Design review of the part built by this model. Coordinates are the model's own, in mm. Face numbers are marked on the shaded views. A direction names the side the tool comes from. Round coordinates to 2 decimals unless told otherwise and drop trailing zeros. Order: outer loops, then holes, each group sorted by start corner. A loop starts at its lowest first (then second) coordinate and runs counter-clockwise, first axis right, second up. Notation, with made-up numbers: (62.5, 89) - (110.5, 89) arc R37 ccw to (110.5, 127) - close; hole circle Ø2 at (75.5, 62.25). An arc over 180 degrees is marked (long way). Use CSV: the item, a comma, the result in double quotes.
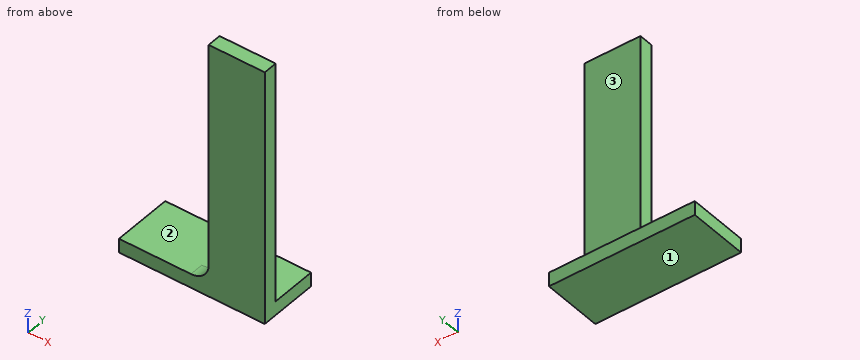
from build123d import *

# Parameters (mm, degrees)
SKETCH1_W      = 52
SKETCH1_H      = 21.25
EXTRUDE1_DEPTH = 5
SKETCH2_W      = 20
SKETCH2_H      = 5
EXTRUDE2_DEPTH = 86.5
FILLET1_R      = 6.35


with BuildPart() as part:
    # Sketch1 → Extrude1 (new body)
    with BuildSketch(Plane.XY):
        with Locations((26, -10.625)):
            Rectangle(SKETCH1_W, SKETCH1_H)
    extrude(amount=EXTRUDE1_DEPTH)

    # Sketch2 → Extrude2 (add)
    with BuildSketch(Plane.XY.offset(5)):
        with Locations((42, -18.75)):
            Rectangle(SKETCH2_W, SKETCH2_H)
    extrude(amount=EXTRUDE2_DEPTH)

    # Fillet1
    fillet1_edges = [part.edges().sort_by_distance(p)[0] for p in [
        (32, -18.75, 5),
    ]]
    fillet(fillet1_edges, radius=FILLET1_R)


solid = part.part
1) Insertion check: pin 1 Ø12 at (y, z) = (-14.5, 55.5) entering from -X; pin 2 Ø1.5 at (y, z) = (-16, 9.5) entering from -X; pin 3 Ø1 at (x, y) = (35.5, -7) entering from -Z; pin 4 Ø6.5 at (x, y) = (36, -12.5) entering from +Z. Each pin has a flat end and moves straight along its axis. Give the tip position at first contact, or say it passes through.
Data:
pin 1,"stops at x = 32"
pin 2,"stops at x = 31.46"
pin 3,"stops at z = 0"
pin 4,"stops at z = 5"
2) We need section B-B (x = 22). Give the boundary of the cut face in (y, z), then the cut area to 3 significant figures.
Data:
outline,"(-21.25, 0) - (0, 0) - (0, 5) - (-21.25, 5) - close"
area,"106 mm2"
3) For the marked faces 1, 2 and 3, list the 3-axis set-ups (+Z, -Z, +X, -X, +Y, -Y) from which the entire face can be reached by the end or side of a thin tool; tool diameter is ignored.
Data:
face 1,"-Z, +X, -X, +Y, -Y"
face 2,"+Z, -X, +Y"
face 3,"+Z, +X, -X, +Y"
4) To check wall thickness, follow L1, parallel to Z at x = 33.5, y = -10.5; L2, parallel to Y at x = 48, z = 10.5; L3, parallel to X at y = -18, z = 81. State the ranges of each line that lie inside material, in increasing order. Write a range as from..to.
Data:
L1,"z = 0..5"
L2,"y = -21.25..-16.25"
L3,"x = 32..52"
5) We need section D-D (x = 41). Give the boundary of the cut face in (y, z).
Data:
outline,"(-21.25, 0) - (0, 0) - (0, 5) - (-16.25, 5) - (-16.25, 91.5) - (-21.25, 91.5) - close"
6) We need section A-A (y = -18). Give the boundary of the cut face in (x, z), then the cut area to 3 significant figures.
Data:
outline,"(0, 0) - (52, 0) - (52, 91.5) - (32, 91.5) - (32, 11.35) arc R6.35 cw to (25.65, 5) - (0, 5) - close"
area,"2,000 mm2"
7) We need section C-C (z = 15). Give the boundary of the cut face in (x, y).
Data:
outline,"(32, -21.25) - (52, -21.25) - (52, -16.25) - (32, -16.25) - close"
